from build123d import *

# Parameters (mm, degrees)
SKETCH_1_R                       = 14
EXTRUDE_1_DEPTH                  = 19
SKETCH_2_R                       = 4.5
EXTRUDE_2_DEPTH                  = 1.5
SKETCH_3_R                       = 4
CUT_EXTRUDE_1_DEPTH              = 1.5
EXTRUDE_START                    = -0.5
EXTRUDE_3_DEPTH                  = 0.5
SKETCH_5_R                       = 2
CUT_EXTRUDE_2_DEPTH              = 32.628019629
EXTRUDE_START_2                  = -15
EXTRUDE_4_DEPTH                  = 15
FILLET_1_R                       = 1
CUT_EXTRUDE_3_DEPTH              = 1
FILLET_2_R                       = 0.3
PATTERN_CIRCULAR_1_COUNT         = 8
FILLET_2_OF_PATTERN_CIRCULAR_1_R = 0.3


with BuildPart() as part:
    # 草图1 → 凸台-拉伸1 (new body)
    with BuildSketch(Plane(origin=(0, 0, 0), x_dir=(1, 0, 0), z_dir=(0, 1, 0))):
        with Locations(Location((0, 0, 0), (0, 0, 270))):
            Circle(SKETCH_1_R)
    extrude(amount=EXTRUDE_1_DEPTH)

    # 草图2 → 凸台-拉伸2 (add)
    with BuildSketch(Plane(origin=(0, 19, 0), x_dir=(1, 0, 0), z_dir=(0, 1, 0))):
        with Locations(Location((0, 8, 0), (0, 0, 270))):
            Circle(SKETCH_2_R)
    extrude(amount=EXTRUDE_2_DEPTH)

    # 草图3 → 切除-拉伸1 (cut)
    with BuildSketch(Plane(origin=(0, 20.5, 0), x_dir=(1, 0, 0), z_dir=(0, 1, 0))):
        with Locations(Location((0, 8, 0), (0, 0, 270))):
            Circle(SKETCH_3_R)
    extrude(amount=-CUT_EXTRUDE_1_DEPTH, mode=Mode.SUBTRACT)

    # 草图4 → 凸台-拉伸3 (add)
    with BuildSketch(Plane(origin=(0, 19, 0), x_dir=(1, 0, 0), z_dir=(0, 1, 0)).offset(EXTRUDE_START)):
        with BuildLine():
            Line((-13.555441712, 3.5), (-17.555441712, 3.5))
            ThreePointArc((-17.555441712, 3.5), (-21.055441712, 0), (-17.555441712, -3.5))
            Line((-17.555441712, -3.5), (-13.555441712, -3.5))
            ThreePointArc((-13.555441712, -3.5), (-14, 0), (-13.555441712, 3.5))
        make_face()
        with BuildLine():
            Line((13.555441712, 3.5), (17.555441712, 3.5))
            ThreePointArc((17.555441712, 3.5), (21.055441712, 0), (17.555441712, -3.5))
            Line((17.555441712, -3.5), (13.555441712, -3.5))
            ThreePointArc((13.555441712, -3.5), (14, 0), (13.555441712, 3.5))
        make_face()
    extrude(amount=EXTRUDE_3_DEPTH)

    # 草图5 → 切除-拉伸2 (cut, through all)
    with BuildSketch(Plane(origin=(0, 19, 0), x_dir=(1, 0, 0), z_dir=(0, 1, 0))):
        with Locations(Location((-17.555441712, 0, 0), (0, 0, 270))):
            Circle(SKETCH_5_R)
        with Locations(Location((17.555441712, 0, 0), (0, 0, 90))):
            Circle(SKETCH_5_R)
    extrude(amount=-CUT_EXTRUDE_2_DEPTH, mode=Mode.SUBTRACT)

    # 草图6 → 凸台-拉伸4 (add)
    with BuildSketch(Plane(origin=(0, 19, 0), x_dir=(1, 0, 0), z_dir=(0, 1, 0)).offset(EXTRUDE_START_2)):
        with BuildLine():
            Line((-6, -12.649110641), (-6, -15.649110641))
            Line((-6, -15.649110641), (6, -15.649110641))
            Line((6, -15.649110641), (6, -12.649110641))
            ThreePointArc((6, -12.649110641), (0, -14), (-6, -12.649110641))
        make_face()
    extrude(amount=EXTRUDE_4_DEPTH)

    # 圆角1
    fillet_1_edges = [part.edges().sort_by_distance(p)[0] for p in [
        (0, 0, -14),
    ]]
    fillet(fillet_1_edges, radius=FILLET_1_R)

    # 草图7 → 切除-拉伸3 (cut)
    with BuildSketch(Plane.XZ):
        with BuildLine():
            Line((0.697808785, 4.951066845), (2.97689197, 8.493415932))
            ThreePointArc((2.97689197, 8.493415932), (3.444150891, 8.314915793), (3.900771502, 8.1107325))
            Line((3.900771502, 8.1107325), (3.007507616, 3.994358264))
            ThreePointArc((3.007507616, 3.994358264), (1.913417162, 4.619397663), (0.697808785, 4.951066845))
        make_face()
    cut_extrude_3 = extrude(amount=-CUT_EXTRUDE_3_DEPTH, mode=Mode.SUBTRACT)

    # 圆角2
    fillet_2_edges = [part.edges().sort_by_distance(p)[0] for p in [
        (2.97689197, 0.5, 8.493415932),
        (3.900771502, 0.5, 8.1107325),
    ]]
    fillet(fillet_2_edges, radius=FILLET_2_R)

    # 阵列(圆周)1: 切除-拉伸3 ×8 about axis
    pattern_circular_1_axis = Axis((-0.034019588, 0, -0.082130551), (0, 1, 0))
    for i in range(1, PATTERN_CIRCULAR_1_COUNT):
        add(cut_extrude_3.rotate(pattern_circular_1_axis, i * 360 / PATTERN_CIRCULAR_1_COUNT), mode=Mode.SUBTRACT)

    # 圆角2 of 阵列(圆周)1
    fillet_2_of_pattern_circular_1_edges = [part.edges().sort_by_distance(p)[0] for p in [
        (8.158843463, 0.5, 3.85266054),
        (8.541526895, 0.5, 2.928781007),
        (8.541526895, 0.5, -3.093042109),
        (8.158843463, 0.5, -4.016921641),
        (3.900771502, 0.5, -8.274993601),
        (2.97689197, 0.5, -8.657677034),
        (-3.044931146, 0.5, -8.657677034),
        (-3.968810678, 0.5, -8.274993601),
        (-8.226882639, 0.5, -4.016921641),
        (-8.609566071, 0.5, -3.093042109),
        (-8.609566071, 0.5, 2.928781007),
        (-8.226882639, 0.5, 3.85266054),
        (-3.968810678, 0.5, 8.1107325),
        (-3.044931146, 0.5, 8.493415932),
    ]]
    fillet(fillet_2_of_pattern_circular_1_edges, radius=FILLET_2_OF_PATTERN_CIRCULAR_1_R)


solid = part.part
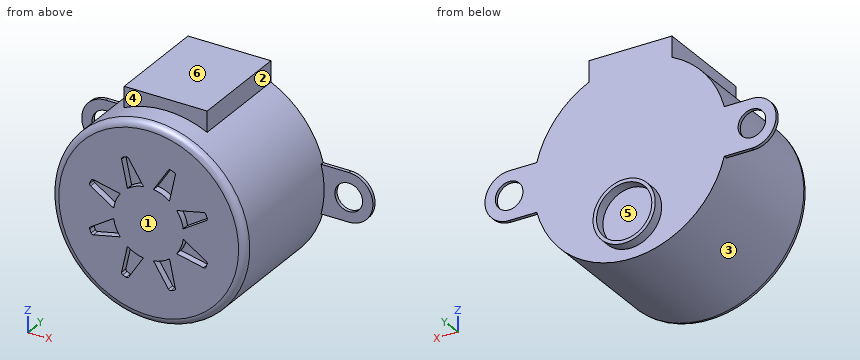
Could you check a few things on this model? Use its own coordinates, in mm. Face numbers are marked on the shaded views. A direction names the side the tool comes from. Coordinates: 2 decimals unless noted, no trailing zeros. Order: outer loops, then holes, each group sorted by start corner. A loop starts at its lowest first (then second) coordinate and runs counter-clockwise, first axis right, second up. Notation, with made-up numbers: (41.25, 26) - (64.25, 26) arc R25 cw to (64.25, 62) - close; hole circle Ø10 at (12.25, -30). An arc over 180 degrees is marked (long way). Answer in a Markdown table with one row per item. Add a question column.
(1) If we mould it in two halves opening along Z, with no side actions, what happens to the marked faces 4, 5 and 6? For each: released by +Z, released by -Z, zero draft, split by the parting line, or undercut.
(2) If we section it at B-B, the plane x = 0: Please give me the cut outline in (y, z), then the cut area to 3 significant figures.
(3) If we section it at A-A, the plane z = 0: Please give me the cut outline in (x, y).
(4) If we section it at D-D, the plane y = 3.5: Please give me the cut outline in (x, z).
(5) Will these pins go through, and if not, where does the flat tip stop? pin 1 (5 mm diameter, centred on y = 2, z = 12.5, fed in from +X); pin 2 (2.5 mm diameter, centred on x = -1.5, z = -6.5, fed in from +Y); pin 3 (3 mm diameter, centred on y = 8, z = -8, fed in from +X); pin 4 (3.5 mm diameter, centred on x = 17.56, z = 0, fed in from -Y).
(6) I need wall thicknesses on L1, parallel to X at y = 18.7, z = 0; L2, parallel to X at y = 19.6, z = -8; L3, parallel to Y at x = 3, z = -7.25. Which ranges of each line are inside material? Lowest first, please.
(7) On a 3-axis mill with a long thin cutter (end or side, diameter ignored), from which of +Z, -Z, +X, -X, +Y, -Y can I reach the whole of each face in a straight line? I mean the marked faces 1, 2 and 3. Say none if no direction works.
(8) If we section it at C-C, the plane x = 16: Please give me the cut outline in (y, z).
Results are:
| question | item | result |
|---|---|---|
| 1 | face 4 | zero draft |
| 1 | face 5 | undercut |
| 1 | face 6 | released by +Z |
| 2 | outline | (0, -13) arc R1 ccw to (1, -14) - (19, -14) - (19, -12.5) - (20.5, -12.5) - (20.5, -12) - (19, -12) - (19, -4) - (20.5, -4) - (20.5, -3.5) - (19, -3.5) - (19, 15.65) - (4, 15.65) - (4, 14) - (1, 14) arc R1 ccw to (0, 13) - close |
| 2 | area | 558 mm2 |
| 3 | outline | (-21.06, 18.5) - (-19.56, 18.5) - (-19.56, 19) - (-21.06, 19) - close; (-15.56, 18.5) - (-14, 18.5) - (-14, 1) arc R1 ccw to (-13, 0) - (13, 0) arc R1 ccw to (14, 1) - (14, 18.5) - (15.56, 18.5) - (15.56, 19) - (-15.56, 19) - close; (19.56, 18.5) - (21.06, 18.5) - (21.06, 19) - (19.56, 19) - close |
| 4 | outline | circle Ø28 at (0, 0) |
| 5 | pin 1 | stops at x = 9.8 |
| 5 | pin 2 | stops at y = 19 |
| 5 | pin 3 | stops at x = 12.4 |
| 5 | pin 4 | passes through |
| 6 | L1 | x = -21.06 to -19.56, -15.56 to 15.56, 19.56 to 21.06 |
| 6 | L2 | x = -4.5 to -4, 4 to 4.5 |
| 6 | L3 | y = 1 to 19 |
| 7 | face 1 | +Z, -Z, +X, -X, -Y |
| 7 | face 2 | +Z, +X, +Y, -Y |
| 7 | face 3 | -Y |
| 8 | outline | (18.5, -3.5) - (19, -3.5) - (19, -1.26) - (18.5, -1.26) - close; (18.5, 1.26) - (19, 1.26) - (19, 3.5) - (18.5, 3.5) - close |
